For this review, take the finished solid that the model builds, in its own axes (mm). A direction names the side the tool comes from. Round coordinates to 2 decimals unless told otherwise and drop trailing zeros. Loops run counter-clockwise (first coordinate to the right, second up) from the corner with the lowest first, then second, coordinate; pieces in that order, holes last. Notation, with made-up numbers: M -23.75,6.5 L 25.25,6.5 A18 cw 25.25,25.5 Z; hole C -2.75,70.25 d11. An arc over 180 degrees is marked long. Write item = value, one per line. Start each with the question number.
Autodesk Inventor part; units mm, degrees
ref_plane "Work Plane1" through (25, 7.0504, 11.25) normal (0, 0, 1) x (1, 0, 0)
ref_plane "YZ Plane" through (0, 0, 0) normal (1, 0, 0) x (0, 1, 0)
ref_plane "XZ Plane" through (0, 0, 0) normal (0, 1, 0) x (-1, 0, 0)
sketch "Sketch1" plane through (0, 0, 0) normal (0, 0, 1) x (1, 0, 0)
  line L0 (-39.25, 1) -> (39.25, 1)
  line L1 (39.25, 1) -> (39.25, -1)
  line L2 (39.25, -1) -> (-39.25, -1)
  line L3 (-39.25, -1) -> (-39.25, 1)
  circle A0 centre (-36.63, 3.5) radius 1.5
  circle A1 centre (28.75, 3.875) radius 1.5
  line L4 (39.25, 6.75) -> (38, 6.75)
  line L5 (38, 6.75) -> (38, 26.75)
  line L6 (38, 26.75) -> (-38, 26.75)
  line L7 (-38, 26.75) -> (-38, 6.75)
  line L8 (-38, 6.75) -> (-39.25, 6.75)
  line L9 (-39.25, 6.75) -> (-39.25, 1)
  line L10 (-39.25, 1) -> (39.25, 1)
  line L11 (39.25, 6.75) -> (39.25, 1)
  line L12 (-34.38, 1) -> (-38.88, 1)
  line L13 (-38.88, 1) -> (-38.88, 3.5)
  line L14 (-38.88, 3.5) -> (-34.38, 3.5)
  line L15 (-34.38, 3.5) -> (-34.38, 1)
  arc A2 (-34.38, 3.5) -> (-38.88, 3.5) centre (-36.63, 3.5) ccw
  line L16 (31, 1) -> (26.5, 1)
  line L17 (26.5, 1) -> (26.5, 3.875)
  line L18 (26.5, 3.875) -> (31, 3.875)
  line L19 (31, 3.875) -> (31, 1)
  arc A3 (31, 3.875) -> (26.5, 3.875) centre (28.75, 3.875) ccw
  line L20 (31.5, 5.4627) -> (31.5, 2.2873)
  line L21 (31.5, 2.2873) -> (28.75, 0.6996)
  line L22 (28.75, 0.6996) -> (26, 2.2873)
  line L23 (26, 2.2873) -> (26, 5.4627)
  line L24 (26, 5.4627) -> (28.75, 7.0504)
  line L25 (28.75, 7.0504) -> (31.5, 5.4627)
  line L26 (32.5, 1) -> (25, 1)
  line L27 (25, 1) -> (25, 7.0504)
  line L28 (25, 7.0504) -> (32.5, 7.0504)
  line L29 (32.5, 7.0504) -> (32.5, 1)
  point P0 (0, 0)
  point P1 (0, 1)
  point P2 (39.25, 0)
  point P3 (0, 35)
  point P4 (28.75, 7.0504)
  dimension "d0" = 2
  dimension "d1" = 78.5
  dimension "d4" = 2.62
  dimension "d5" = 2.5
  dimension "d6" = 3
  dimension "d7" = 4.5
  dimension "d8" = 2.875
  dimension "d9" = 10.5
  dimension "d10" = 3
  dimension "d11" = 4.5
  dimension "d12" = 5.5
  dimension "d13" = 7.5
  dimension "d14" = 0
extrude "Extrusion1" add sketch "Sketch1" along normal blind 22.5 contours L0 L22 L21 L1 L2 L3 | L13 L14 A0 L15 L0 | A2 L14 A0 | L27 L28 L24 L23 L22 L17 L0 | L17 L22 L0 | L0 L19 L21 L20 L25 L28 L29 | L22 L17 L18 A1 L19 L21 L0 | L0 L21 L22 | L22 L23 L24 L25 L20 L21 L19 A3 L17 | L0 L21 L19 | A3 L18 A1
sketch "Sketch2" plane through (39.25, -1, 0) normal (1, 0, 0) x (0, 0, -1)
  line L0 (-22.5, 0) -> (-22.5, 2)
  line L1 (0, 8.0504) -> (-22.5, 8.0504)
  line L2 (-22.5, 2) -> (-18, 2)
  line L3 (-18, 2) -> (-18, 8.0504)
  line L4 (-18, 8.0504) -> (-22.5, 8.0504)
  line L5 (-22.5, 8.0504) -> (-22.5, 2)
  line L6 (-18, 2) -> (-13.5, 2)
  line L7 (-13.5, 2) -> (-13.5, 8.0504)
  line L8 (-13.5, 8.0504) -> (-18, 8.0504)
  line L9 (-18, 8.0504) -> (-18, 2)
  line L10 (0, 2) -> (-22.5, 2)
  line L11 (-4.5, 2) -> (-9, 2)
  line L12 (-9, 2) -> (-9, 8.0504)
  line L13 (-9, 8.0504) -> (-4.5, 8.0504)
  line L14 (-4.5, 8.0504) -> (-4.5, 2)
  line L15 (0, 2) -> (-4.5, 2)
  line L16 (-4.5, 2) -> (-4.5, 8.0504)
  line L17 (-4.5, 8.0504) -> (0, 8.0504)
  line L18 (0, 8.0504) -> (0, 2)
  line L19 (-9, 8.0504) -> (-13.5, 8.0504)
  line L20 (-13.5, 8.0504) -> (-13.5, 2)
  line L21 (-13.5, 2) -> (-9, 2)
  line L22 (-9, 2) -> (-9, 8.0504)
  point P0 (0, 1)
  dimension "d15" = 4.5
  dimension "d16" = 4.5
  dimension "d17" = 4.5
  dimension "d18" = 4.5
extrude "Extrusion2" cut sketch "Sketch2" against normal up to surface (14.25 mm away) contours L18 L10 L14 L1 | L12 L10 L7 L1 | L3 L2 L5 L1
sketch "Sketch3" plane through (25, 7.0504, 18) normal (0, 1, 0) x (1, 0, 0)
  line L0 (6.65, 1) -> (0.85, 1)
  line L1 (0.85, 1) -> (0.85, 3.5)
  line L2 (0.85, 3.5) -> (6.65, 3.5)
  line L3 (6.65, 3.5) -> (6.65, 1)
  line L4 (0, 0) -> (7.5, 0)
  line L5 (7.5, 4.5) -> (7.5, 0)
  line L6 (6.65, 10) -> (0.85, 10)
  line L7 (0.85, 10) -> (0.85, 12.5)
  line L8 (0.85, 12.5) -> (6.65, 12.5)
  line L9 (6.65, 12.5) -> (6.65, 10)
  line L10 (0, 9) -> (7.5, 9)
  line L11 (7.5, 13.5) -> (7.5, 9)
  point P0 (-25, 18)
  point P1 (3.75, 1)
  point P2 (3.75, 0)
  point P3 (6.65, 2.25)
  point P4 (7.5, 2.25)
  point P5 (3.75, 10)
  point P6 (3.75, 9)
  point P7 (6.65, 11.25)
  point P8 (7.5, 11.25)
  dimension "d21" = 5.8
  dimension "d22" = 2.5
  dimension "d23" = 5.8
  dimension "d24" = 2.5
extrude "Extrusion3" cut sketch "Sketch3" against normal blind 6.351
sketch "Sketch4" plane through (25.85, 7.0504, 5.5) normal (0, 0, 1) x (1, 0, 0)
  circle A0 centre (2.9, -3.1754) radius 1.5
  line L0 (0, 0) -> (5.8, 0)
  line L1 (0, 0) -> (0, -6.351)
  line L2 (0, -6.351) -> (5.8, -6.351)
  line L3 (5.8, 0) -> (5.8, -6.351)
  line L4 (2.9, -6.351) -> (0, -4.6767)
  line L5 (0.1499, -4.7632) -> (0.1499, -1.5876)
  line L6 (0.1499, -1.5876) -> (2.9, 0.0001)
  line L7 (2.9, 0.0001) -> (5.6501, -1.5876)
  line L8 (5.6501, -1.5876) -> (5.6501, -4.7632)
  line L9 (5.8, -4.6767) -> (2.9, -6.351)
  point P0 (-25.85, -7.0504)
extrude "Extrusion4" add sketch "Sketch4" along normal up to surface (2.5 mm away) contours L4 L2 L1 | L3 L2 L9
ref_plane "Work Plane1" through (25, 7.0504, 11.25) normal (0, 0, 1) x (1, 0, 0)
mirror "Mirror1" about plane through (25, 7.0504, 11.25) normal (0, 0, 1) of "Extrusion4"
sketch "Sketch5" plane through (-39.25, -1, 0) normal (0, -1, 0) x (1, 0, 0)
  line L0 (6.1251, 17.7549) -> (72.3749, 17.7549) construction
  line L1 (72.3749, 17.7549) -> (72.3749, 4.7451) construction
  line L2 (72.3749, 4.7451) -> (6.1251, 4.7451) construction
  line L3 (6.1251, 4.7451) -> (6.1251, 17.7549) construction
  line L4 (0, 22.5) -> (78.5, 22.5)
  line L5 (78.5, 0) -> (78.5, 22.5)
  point P0 (39.25, 0)
  point P1 (39.25, 17.7549)
  point P2 (39.25, 22.5)
  point P3 (72.3749, 11.25)
  point P4 (78.5, 11.25)
sketch "Sketch6" plane through (-39.25, -1, 0) normal (-1, 0, 0) x (0, 0, 1)
  line L0 (0, 0) -> (0, 2)
  line L1 (0, 6.75) -> (22.5, 6.75)
  line L2 (0, 2) -> (1.5, 2)
  line L3 (1.5, 2) -> (1.5, 6.75)
  line L4 (1.5, 6.75) -> (0, 6.75)
  line L5 (0, 6.75) -> (0, 2)
  point P0 (0, 1)
  dimension "d30" = 1.5
extrude "Extrusion5" cut sketch "Sketch6" against normal blind 10
equation "\"d11\" = d7"
equation "\"d17\" = d15"
equation "\"d18\" = d16"
equation "\"d23\" = d21"
equation "\"d24\" = d22"
properties part number "vrata"
(1) Wall thickness on L1, parallel to X at y = 3.5, z = 10.25; L2, parallel to X at y = 4.75, z = 16.75; L3, parallel to Y at x = 28.75, z = 5.15 (3 decimals): over which ranges is each line inside the solid? List them lowest first.
(2) Add section C-C on x = 28. Count the separate pieces of the cut face and the enclosed holes in it, and give its area (3 significant figures).
(3) Add section B-B on z = 10.5. Write out the cut boundary in (x, y), and give its area (3 significant figures).
(4) Draft analysis for pull direction X (two halves, no side actions). For faces 6 (the flat face through (-38.88, 2, 12)), 7 (the cylindrical face through (-38.13, 3.43, 11.85)), 8 (the flat face through (1, -1, 11)), state which applies: +X half, -X half, draft (parallel to the pull), parting line (faces both ways), or undercut.
(5) Add section A-A on x = -36.63. Write out the cut boundary in (y, z).
(6) Tool access review of faces 1 (the flat face through (27.28, 1.55, 15.77)), 2 (the flat face through (30, 5, 18)), 3 (the flat face through (28.7, 7.05, 8.2)), 4 (the flat face through (32.5, 4, 16)), 5 (the flat face through (30, 5, 4.5)): name each direction out of +Z, -Z, +X, -X, +Y, -Y from which nothing blocks a thin tool from reaching the whole face with its end or side.
(7) For pin 1 Ø2 at (y, z) = (5.5, 15.5) entering from -X; pin 2 Ø2.5 at (x, y) = (28.75, 3.875) entering from -Z; pin 3 Ø2 at (x, y) = (-37, 4) entering from -Z; pin 4 Ø4.5 at (x, y) = (30, 3.5) entering from +Z, all flat-tipped, find the tip position at first contact; note any pin that passes through.
Answer sheet:
q1.L1 = -38.88 to -38.13, -35.13 to -34.38
q1.L2 = -38.5 to -37.46, -35.8 to -34.76, 25 to 25.85, 31.65 to 32.5
q1.L3 = -1 to 2.375, 5.375 to 7.05
q2.separate_pieces = 5
q2.enclosed_holes = 0
q2.area = 59.5 mm²
q3.outline = M -39.25,-1 L 39.25,-1 L 39.25,1 L -34.38,1 L -34.38,3.5 A2.25 ccw -38.88,3.5 L -38.88,1 L -39.25,1 Z; hole C -36.63,3.5 d3
q3.area = 169 mm²
q4.face_6 = -X half
q4.face_7 = undercut
q4.face_8 = draft
q5.outline = M -1,0 L 1,0 L 1,1.5 L 2,1.5 L 2,22.5 L -1,22.5 Z; M 5,1.5 L 5.75,1.5 L 5.75,22.5 L 5,22.5 Z
q6.face_1 = +Y
q6.face_2 = +Z, +X, +Y
q6.face_3 = +Z, -Z, +X, -X, +Y
q6.face_4 = +Z, -Z, +X, +Y
q6.face_5 = -Z, +X, +Y
q7.pin_1 = -38.65
q7.pin_2 = through
q7.pin_3 = 1.5
q7.pin_4 = 18
